```python
from build123d import *

# Parameters (mm, degrees)
F0_W      = 69.25
F0_H      = 19.25
F1_DEPTH  = 8.5
F3_SIZE2  = 1
F3_SIZE   = 3.5
F4_SIZE2  = 4.99999
F4_SIZE   = 1.99999
F2_W      = 64
F2_H      = 15.5
F5_DEPTH  = 7
F6_W      = 52
F6_H      = 12.2
F7_DEPTH  = 2
F8_W      = 7.9
F8_H      = 7.7
F8_H_2    = 2.2
F9_DEPTH  = 2
F8_W_2    = 13.4
F8_H_3    = 5.4
F10_DEPTH = 25
F11_W     = 50
F11_H     = 8.2
F11_W_2   = 13.4
F11_H_2   = 5.4
F11_H_3   = 5.3
F12_DEPTH = 1.5
F13_SIZE  = 1.5


# Not quite as in the source:
# - a fillet or chamfer is up to 0.001 mm smaller than in the source, because OpenCascade refuses the exact size


with BuildPart() as f1:
    # F0 (on Top) → F1 (new body)
    with BuildSketch(Plane.XY):
        Rectangle(F0_W, F0_H)
    extrude(amount=F1_DEPTH)

    # F3
    f3_edges = [f1.edges().sort_by_distance(p)[0] for p in [
        (-34.625, 0, 8.5),
        (0, -9.625, 8.5),
        (34.625, 0, 8.5),
        (0, 9.625, 8.5),
    ]]
    chamfer(f3_edges, length=F3_SIZE, length2=F3_SIZE2)

    # F4 (size 2 and 5 in the source; OpenCascade refuses exactly that, so slightly less here)
    f4_edges = [f1.edges().sort_by_distance(p)[0] for p in [
        (-34.625, 0, 0),
        (0, -9.625, 0),
        (0, 9.625, 0),
        (34.625, 0, 0),
    ]]
    f4_side = f1.faces().sort_by_distance((0, 0, 0))[0]
    chamfer(f4_edges, length=F4_SIZE, length2=F4_SIZE2, reference=f4_side)

    # F2 (on face) → F5 (cut)
    with BuildSketch(Plane.XY.offset(8.5)):
        Rectangle(F2_W, F2_H)
    extrude(amount=-F5_DEPTH, mode=Mode.SUBTRACT)

    # F6 (on face) → F7 (join)
    with BuildSketch(Plane(origin=(0, 0, 0), x_dir=(1, 0, 0), z_dir=(0, 0, -1))):
        Rectangle(F6_W, F6_H)
    extrude(amount=F7_DEPTH)

    # F8 (on face) → F9 (cut)
    with BuildSketch(Plane(origin=(0, 0, -2), x_dir=(1, 0, 0), z_dir=(0, 0, -1))):
        with Locations((0, -1.1)):
            Rectangle(F8_W, F8_H)
        with Locations((0, 3.85)):
            Rectangle(F8_W, F8_H_2)
    extrude(amount=-F9_DEPTH, mode=Mode.SUBTRACT)

    # F8 (on face) → F10 (cut)
    with BuildSketch(Plane(origin=(0, 0, -2), x_dir=(1, 0, 0), z_dir=(0, 0, -1))):
        with Locations((-15.9, 0.05)):
            Rectangle(F8_W_2, F8_H_3)
        Polygon((15.7195143402, 2.75), (9.2, 2.75), (9.2, -2.55), (22.6, -2.55), (22.6, 2.75), align=None)
    extrude(amount=-F10_DEPTH, mode=Mode.SUBTRACT)

    # F11 (on face) → F12 (cut)
    with BuildSketch(Plane.XY.offset(1.5)):
        Rectangle(F11_W, F11_H)
        with Locations((-15.9, -0.05)):
            Rectangle(F11_W_2, F11_H_2, mode=Mode.SUBTRACT)
        with Locations((15.9, -0.1)):
            Rectangle(F11_W_2, F11_H_3, mode=Mode.SUBTRACT)
    extrude(amount=-F12_DEPTH, mode=Mode.SUBTRACT)

    # F13
    f13_edges = [f1.edges().sort_by_distance(p)[0] for p in [
        (-32, 0, 1.5),
        (0, 7.75, 1.5),
        (32, 0, 1.5),
        (0, -7.75, 1.5),
    ]]
    chamfer(f13_edges, length=F13_SIZE)


solid = f1.part
```
Here's how the part is built. I have some questions about the finished solid (model axes, mm). A direction names the side the tool comes from. Give positions to 0.01 mm unless a question says otherwise; leave off trailing zeros. Order: outer loops, then holes, each group sorted by start corner. A loop starts at its lowest first (then second) coordinate and runs counter-clockwise, first axis right, second up. Notation, with made-up numbers: M 31.5,6.5 L 36.5,6.5 A16 ccw 36.5,22.5 Z; hole C 39.5,0 d7. An arc over 180 degrees is marked long. Use a Markdown table: item, result. Add a question column.
1. For pin 1 Ø1 at (x, z) = (-1.5, -1) entering from +Y; pin 2 Ø1 at (y, z) = (0.5, -1) entering from -X; pin 3 Ø1.6 at (y, z) = (-1.5, 1) entering from +X (3 decimals), each with a flat end and sliding along its axis, tell me the tip position at first contact or that it passes through.
2. If we mould it in two halves opening along X, with no side actions, what happens to faces 1 (the flat face through (-34.12, -0.13, 6.77)), 2 (the flat face through (26, 0, -1)), 3 (the flat face through (0, 4.1, 1)), 4 (the flat face through (-0.485, 8.639, 2.535))? For each: +X half, -X half, draft (parallel to the pull), parting line (faces both ways), or undercut.
3. I need wall thicknesses on probe 1 along X at (y, z) = (1.25, -1); probe 2 along Z at (x, y) = (-19, -5); probe 3 along Y at (x, z) = (-9, 6.5). Which ranges of each line are inside material? Lowest first, please. Write a range as from..to.
4. On a 3-axis mill with a long thin cutter (end or side, diameter ignored), from which of +Z, -Z, +X, -X, +Y, -Y can I reach the whole of each face in a straight line? I mean faces 5 (the flat face through (22.6, 0, -1)), 6 (the flat face through (-25, 0, 1)), 7 (the flat face through (0, 4.95, -1)), 8 (the flat face through (0, 6.1, -1)). Say none if no direction works.
5. Suppose I cut it at C-C (z = 4.25). List the corners of the cut face in (x, y) for me (3 decimals).
6. Suppose I cut it at A-A (y = 0.5). Give the number of separate pieces and of enclosed holes in the cut face, and give its area (3 significant figures).
Results list:
| question | item | result |
|---|---|---|
| 1 | pin 1 | stops at y = 6.1 |
| 1 | pin 2 | stops at x = -26 |
| 1 | pin 3 | stops at x = 33.345 |
| 2 | face 1 | -X half |
| 2 | face 2 | +X half |
| 2 | face 3 | undercut |
| 2 | face 4 | draft |
| 3 | probe 1 | x = -26..-22.6, -9.2..-3.95, 3.95..9.2, 22.6..26 |
| 3 | probe 2 | z = -2..1.5 |
| 3 | probe 3 | y = -9.2..-7.75, 7.75..9.2 |
| 4 | face 5 | +Z, -Z |
| 4 | face 6 | +Z |
| 4 | face 7 | -Z |
| 4 | face 8 | -Z, +X, -X, +Y |
| 5 | outline | M -34.325,-9.325 L 34.325,-9.325 L 34.325,9.325 L -34.325,9.325 Z; hole M -32,-7.75 L 32,-7.75 L 32,7.75 L -32,7.75 Z |
| 6 | separate pieces | 4 |
| 6 | enclosed holes | 0 |
| 6 | area | 89.0 mm² |
